Geometry check sheet. Reference: drawing and pictorial views, mm from the part's lowest x, y, z. Give positions to 0.01 mm unless a question says otherwise; leave off trailing zeros. Loops run counter-clockwise (first coordinate to the right, second up) from the corner with the lowest first, then second, coordinate; pieces in that order, holes last. Notation, with made-up numbers: (-29, 64.25) - (-13, 64.25) arc R27 ccw to (-13, 90.25) - close; hole circle Ø8 at (51, 62). An arc over 180 degrees is marked (long way). Put each result on its own line as item: value. Start each with the question number.
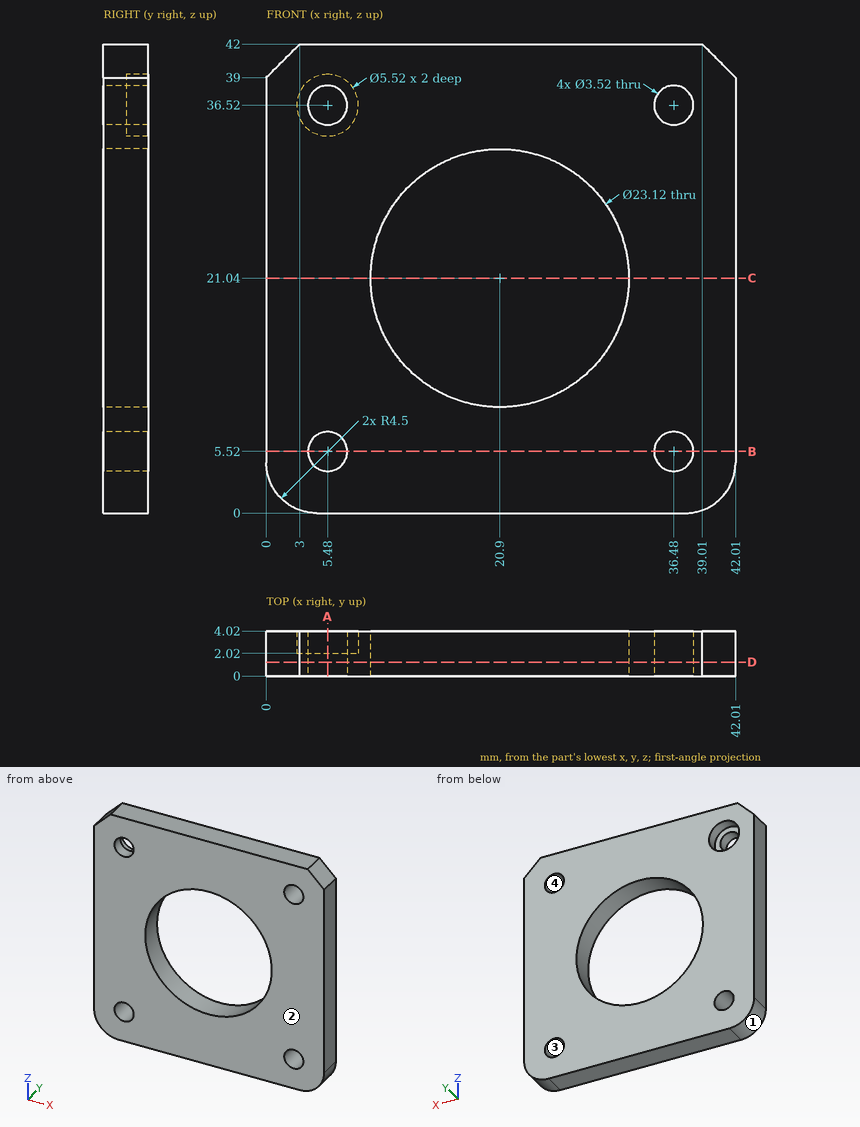
1) Scan lines: line 1 along X through (y, z) = (2.25, 5.52); line 2 along Z through (x, y) = (5.48, 0.8); line 3 along X through (y, z) = (3.85, 5). Record each from-to range of solid material in increasing order. Write a range as from..to.
2) Section check C-C, the plane z = 21.04. Enter the section's corners in (x, y).
3) Section check B-B, the plane z = 5.52. Enter the section's corners in (x, y), plus the area to 3 significant figures.
4) Draft check along X on the marked faces 1, 2, 3 and 4. Enter one of: pulls with the +X half, pulls with the -X half, needs draft (parallel to the pull), parting line crosses it, or undercut.
5) Section check D-D, the plane y = 1.25. Enter the section's corners in (x, z), plus the area to 3 significant figures.
6) Section check A-A, the plane x = 5.48. Enter the section's corners in (y, z), plus the area to 3 significant figures.
Results are:
1. line 1: x = 0..3.72, 7.24..34.72, 38.24..42.01
1. line 2: z = 0..3.76, 7.28..34.76, 38.28..42
1. line 3: x = 0..3.8, 7.16..34.8, 38.16..42.01
2. outline: (0, 0) - (9.34, 0) - (9.34, 4.02) - (0, 4.02) - close; (32.46, 0) - (42.01, 0) - (42.01, 4.02) - (32.46, 4.02) - close
3. outline: (0, 0) - (3.72, 0) - (3.72, 4.02) - (0, 4.02) - close; (7.24, 0) - (34.72, 0) - (34.72, 4.02) - (7.24, 4.02) - close; (38.24, 0) - (42.01, 0) - (42.01, 4.02) - (38.24, 4.02) - close
3. area: 141 mm2
4. face 1: pulls with the -X half
4. face 2: needs draft
4. face 3: undercut
4. face 4: undercut
5. outline: (0, 4.5) arc R4.5 ccw to (4.5, 0) - (37.51, 0) arc R4.5 ccw to (42.01, 4.5) - (42.01, 39) - (39.01, 42) - (3, 42) - (0, 39) - close; hole circle Ø3.52 at (5.48, 5.52); hole circle Ø3.52 at (5.48, 36.52); hole circle Ø23.12 at (20.9, 21.04); hole circle Ø3.52 at (36.48, 5.52); hole circle Ø3.52 at (36.48, 36.52)
5. area: 1,290 mm2
6. outline: (0, 0) - (4.02, 0) - (4.02, 3.76) - (0, 3.76) - close; (0, 7.28) - (4.02, 7.28) - (4.02, 33.76) - (2.02, 33.76) - (2.02, 34.76) - (0, 34.76) - close; (0, 38.28) - (2.02, 38.28) - (2.02, 39.28) - (4.02, 39.28) - (4.02, 42) - (0, 42) - close
6. area: 137 mm2
